Could you check a few things on this drawing? It's one solid part, dimensions in mm from its lowest x, y, z. Coordinates: 2 decimals unless noted, no trailing zeros. Order: outer loops, then holes, each group sorted by start corner. A loop starts at its lowest first (then second) coordinate and runs counter-clockwise, first axis right, second up.
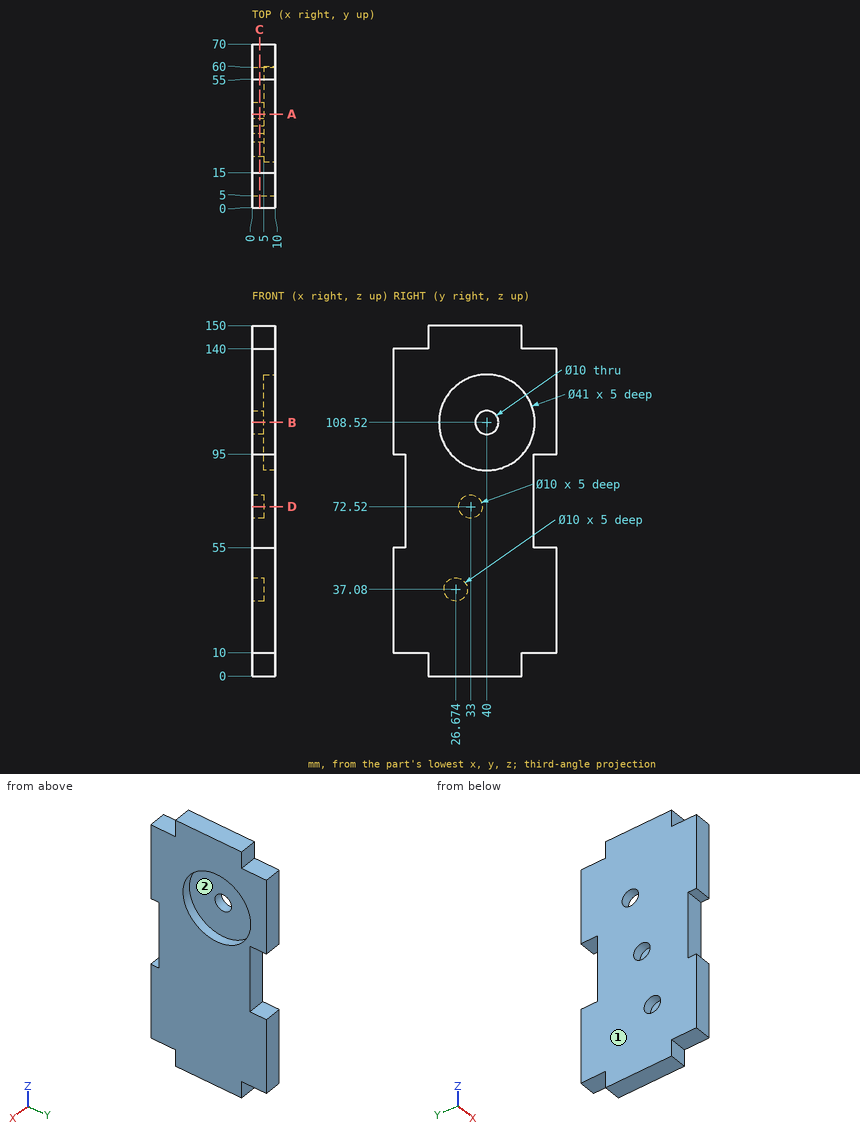
1. I'm going to push flat-ended pins straight in: pin 1 (1.5 mm diameter, centred on x = 2.5, y = 2.5, fed in from -Z); pin 2 (5 mm diameter, centred on x = 7, y = 65, fed in from +Z); pin 3 (5 mm diameter, centred on x = 6, z = 3.5, fed in from +Y). Where does each tip first touch, or does it pass through?
Completed:
pin 1: stops at z = 10
pin 2: stops at z = 140
pin 3: stops at y = 55
2. Imagine slicing it at D-D on z = 72.52. Please give me the cut outline in (x, y), then the cut area to 3 significant figures.
Completed:
outline: (0, 5) - (10, 5) - (10, 60) - (0, 60) - (0, 38) - (5, 38) - (5, 28) - (0, 28) - close
area: 500 mm2
3. Imagine slicing it at A-A on y = 40. Please give me the cut outline in (x, z), then the cut area to 4 significant figures.
Completed:
outline: (0, 0) - (10, 0) - (10, 88.02) - (5, 88.02) - (5, 103.52) - (0, 103.52) - close; (0, 113.52) - (5, 113.52) - (5, 129.02) - (10, 129.02) - (10, 150) - (0, 150) - close
area: 1,245 mm2
4. Imagine slicing it at B-B on z = 108.52. Please give me the cut outline in (x, y), then the cut area to 3 significant figures.
Completed:
outline: (0, 0) - (10, 0) - (10, 19.5) - (5, 19.5) - (5, 35) - (0, 35) - close; (0, 45) - (5, 45) - (5, 60.5) - (10, 60.5) - (10, 70) - (0, 70) - close
area: 445 mm2
5. Imagine slicing it at C-C on x = 3.25. Please give me the cut outline in (y, z) (1 decimal), then the cut area to 3 significant figures.
Completed:
outline: (0, 10) - (15, 10) - (15, 0) - (55, 0) - (55, 10) - (70, 10) - (70, 55) - (60, 55) - (60, 95) - (70, 95) - (70, 140) - (55, 140) - (55, 150) - (15, 150) - (15, 140) - (0, 140) - (0, 95) - (5, 95) - (5, 55) - (0, 55) - close; hole circle Ø10 at (26.7, 37.1); hole circle Ø10 at (33, 72.5); hole circle Ø10 at (40, 108.5)
area: 9,060 mm2
6. Thinking about a two-plate mould opening in Y: for the marked faces 1 and 2, which applies, pulls with the +Y half, pulls with the -Y half, needs draft (parallel to the pull), parting line crosses it, or undercut?
Completed:
face 1: needs draft
face 2: undercut
7. Please list where these lines run through material, in increasing order: probe 1 along Y at (x, z) = (4, 108.52); probe 2 along Z at (x, y) = (6.25, 64.5); probe 3 along Y at (x, z) = (8.25, 108.52).
Completed:
probe 1: y = 0 to 35, 45 to 70
probe 2: z = 10 to 55, 95 to 140
probe 3: y = 0 to 19.5, 60.5 to 70
